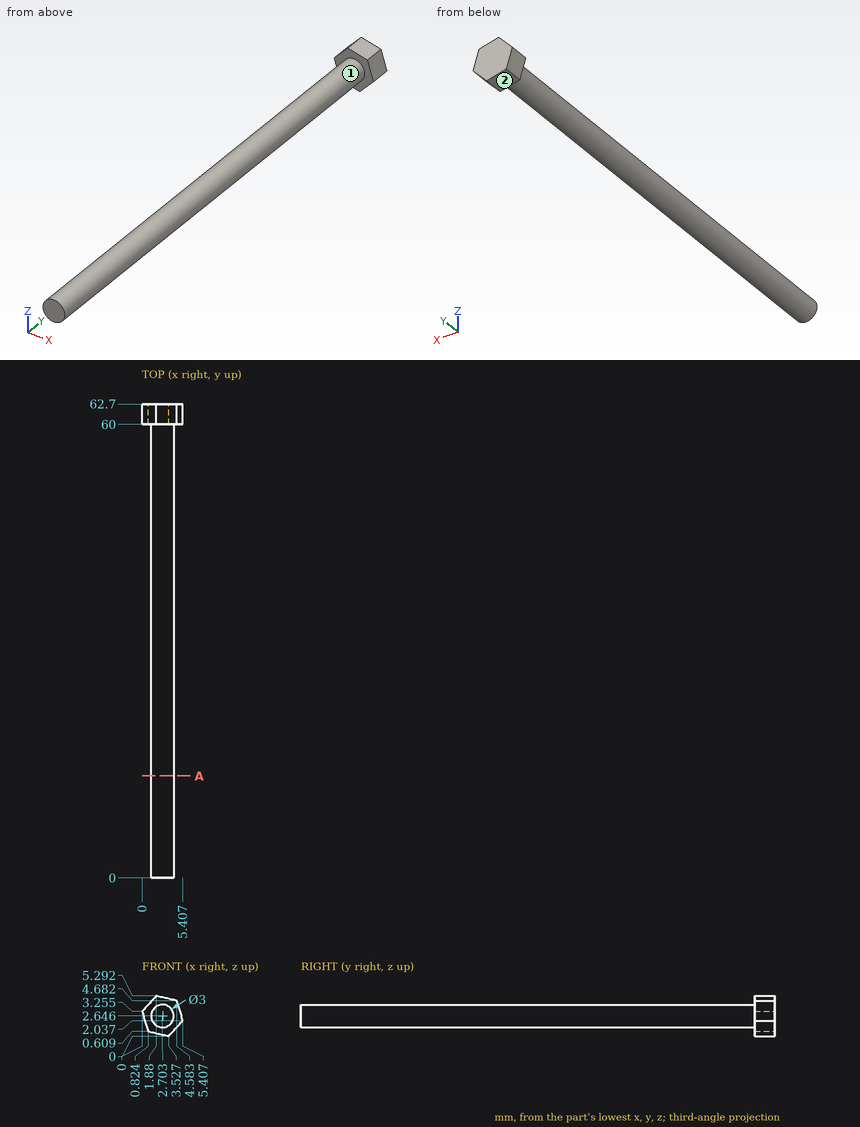
Geometry check sheet. Reference: drawing and pictorial views, mm from the part's lowest x, y, z. A direction names the side the tool comes from. Coordinates: 2 decimals unless noted, no trailing zeros. Order: outer loops, then holes, each group sorted by start corner. A loop starts at its lowest first (then second) coordinate and runs counter-clockwise, first axis right, second up. Notation, with made-up numbers: M 87,63.25 L 132,63.25 A17 cw 132,93.25 Z; hole C 78.25,0.5 d2. An arc over 180 degrees is marked long. Return JSON: item names as keys, results as strings.
1) Access from +Z, -Z, +X, -X, +Y, -Y to the whole of each face (thin tool, end or side, straight path). Record for the marked faces 1 and 2.
Answer list:
{"face 1": "-Y", "face 2": "-Z, -X, +Y, -Y"}
2) Thickness scan on L1, parallel to Y at x = 1.05, z = 3.35; L2, parallel to X at y = 51.5, z = 3.9 (1 decimal); L3, parallel to X at y = 54, z = 2.7 (1 decimal). Record the ranges inside material, lowest first. Write a range as [from, to].
Answer list:
{"L1": "[60, 62.7]", "L2": "[1.9, 3.5]", "L3": "[1.2, 4.2]"}
3) Gauge pin test, flat ends, axial feed: pin 1 (1.5 mm diameter, centred on x = 5, z = 3.5, fed in from -Y); pin 2 (2 mm diameter, centred on x = 1, z = 3, fed in from -Y); pin 3 (3 mm diameter, centred on x = 1, y = 39.5, fed in from -Z); pin 4 (2 mm diameter, centred on x = 0.5, y = 33.5, fed in from +Z). Record the tip position at first contact, or that the pin passes through.
Answer list:
{"pin 1": "y = 60", "pin 2": "y = 0", "pin 3": "z = 1.16", "pin 4": "z = 3.54"}
4) Cross-section at A-A, the plane y = 13.5. Record the boundary of the cut face in (x, z) (1 decimal).
Answer list:
{"outline": "C 2.7,2.6 d3"}
